Build history of the part. All positions in model axes, mm. Round coordinates to 2 decimals unless told otherwise and drop trailing zeros. Write each loop counter-clockwise with the first axis right and the second up, starting at its lowest first coordinate (ties: lowest second). Pieces come first, ordered by that corner, then holes. Notation, with made-up numbers: M -24,78.25 L 7,78.25 A8 ccw 7,90.25 Z; hole C 68.25,-31 d6. An arc over 180 degrees is marked long. Write item = value, one per line.
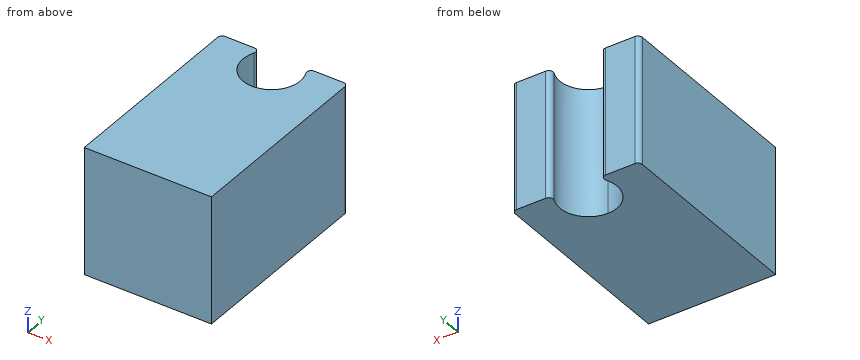
from build123d import *

# Parameters (mm, degrees)
BOSS_EXTRUDE1_DEPTH = 11.1125
SKETCH2_W           = 22.225
SKETCH2_H           = 22.225
BOSS_EXTRUDE2_DEPTH = 1.524


with BuildPart() as part:
    # Sketch1 → Boss-Extrude1 (new body, symmetric)
    with BuildSketch(Plane.XY):
        with BuildLine():
            Line((-11.1125, 2.448544554), (-11.1125, -30))
            Line((-11.1125, -30), (0, -30))
            Line((0, -30), (0, -5))
            ThreePointArc((0, -5), (-4.216957229, -2.686498042), (-4.531538935, 2.113091309))
            ThreePointArc((-4.531538935, 2.113091309), (-4.581478781, 2.875026118), (-5.250920741, 3.242294554))
            Line((-5.250920741, 3.242294554), (-10.31875, 3.242294554))
            ThreePointArc((-10.31875, 3.242294554), (-10.880016008, 3.009810562), (-11.1125, 2.448544554))
        make_face()
    boss_extrude1 = extrude(amount=BOSS_EXTRUDE1_DEPTH, both=True)

    # Mirror1: Boss-Extrude1 across plane
    add(boss_extrude1.mirror(Plane(origin=(0, 0, 0), x_dir=(0, 0, 1), z_dir=(1, 0, 0))))

    # Sketch2 → Boss-Extrude2 (add)
    with BuildSketch(Plane.XZ.offset(30)):
        Rectangle(SKETCH2_W, SKETCH2_H)
    extrude(amount=BOSS_EXTRUDE2_DEPTH)


solid = part.part
1. Band-saw the part on A-A (y = 0). List the corners of the cut face in (x, z), plus the area to 3 significant figures.
Responses:
outline = M -11.11,-11.11 L -5,-11.11 L -5,11.11 L -11.11,11.11 Z; M 5,-11.11 L 11.11,-11.11 L 11.11,11.11 L 5,11.11 Z
area = 272 mm²
2. Band-saw the part on B-B (y = -4). List the corners of the cut face in (x, z).
Responses:
outline = M -11.11,-11.11 L -3,-11.11 L -3,11.11 L -11.11,11.11 Z; M 3,-11.11 L 11.11,-11.11 L 11.11,11.11 L 3,11.11 Z
3. Band-saw the part on D-D (x = 2.5). List the corners of the cut face in (y, z), plus the area to 3 significant figures.
Responses:
outline = M -31.52,-11.11 L -4.33,-11.11 L -4.33,11.11 L -31.52,11.11 Z
area = 604 mm²
4. Probe probe 1 along X at (y, z) = (-2, 7.75); probe 2 along Y at (x, z) = (-0.5, -1.25); probe 3 along Y at (x, z) = (3, 4.25). List the from-to ranges inside material, lowest first.
Responses:
probe_1 = -11.11 to -4.58, 4.58 to 11.11
probe_2 = -31.52 to -4.97
probe_3 = -31.52 to -4
5. Band-saw the part on C-C (z = 0.5). List the corners of the cut face in (x, y).
Responses:
outline = M -11.11,-31.52 L 11.11,-31.52 L 11.11,2.45 A0.79 ccw 10.32,3.24 L 5.25,3.24 A0.79 ccw 4.53,2.11 A5 cw long -4.53,2.11 A0.79 ccw -5.25,3.24 L -10.32,3.24 A0.79 ccw -11.11,2.45 Z
